Geometry: see drawing. Coordinates: mm, zero at the bounding-box minimum. Give positions to 0.01 mm unless a question says otherwise; leave off trailing zeros. Order: outer loops, then holes, each group sorted by start corner. A loop starts at its lowest first (then second) coordinate and runs counter-clockwise, first axis right, second up. Notation, with made-up numbers: (37, 36.5) - (64, 36.5) arc R15 ccw to (64, 50.5) - close; hole circle Ø9 at (79, 18.5). An arc over 180 degrees is marked (long way). Write each question's results on one line, items separated by ' | '. Start each with the question number.
Item 1: Section A-A on y = 33. Output: boundary loops of the cut face in (x, z).
Item 2: Section B-B on x = 77.5. Output: boundary loops of the cut face in (y, z), and give its area (3 significant figures).
Item 3: Section D-D on y = 15.5. Output: boundary loops of the cut face in (x, z), and give its area (3 significant figures).
Item 4: Contact query for flat-ended pins moving along their axis: pin 1 Ø1.5 at (x, z) = (61, 2.5) entering from +Y; pin 2 Ø1.7 at (x, z) = (99.5, 2) entering from +Y (1 decimal); pin 3 Ø1.7 at (x, z) = (2.5, 2.5) entering from +Y. Output: stop coordinate, or through.
Item 5: Line query: line 1 along X through (y, z) = (41, 1); line 2 along X through (y, z) = (63.5, 0.3); line 3 along Y through (x, z) = (50, 2.1) (1 decimal). Output: solid intervals per line, ascending.
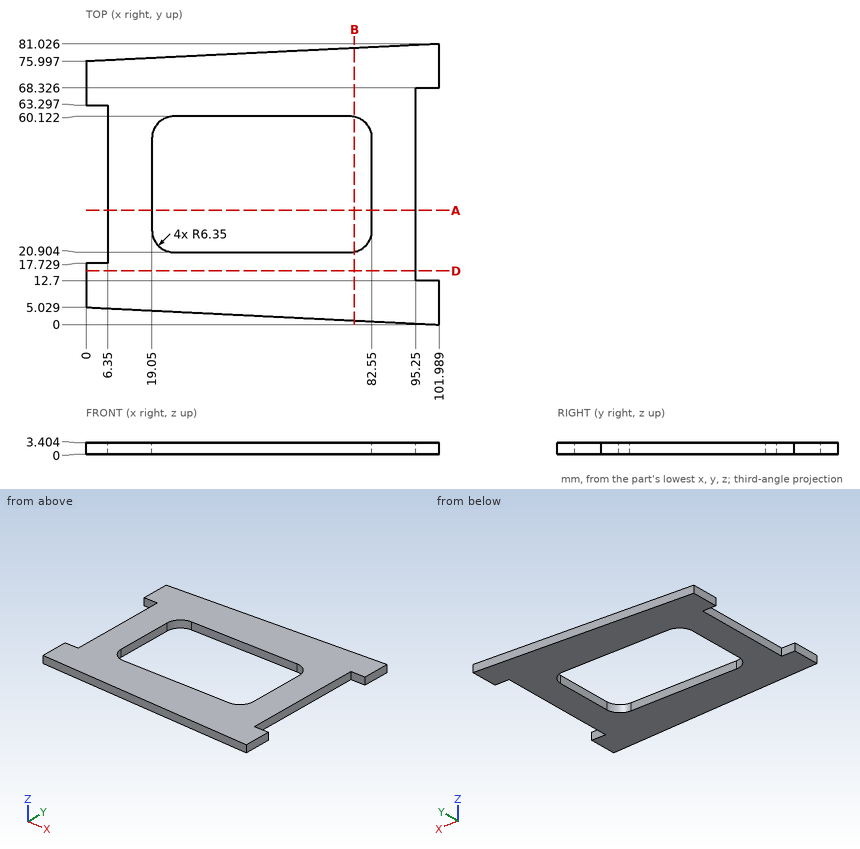
Evaluation:
1) outline: (6.35, 0) - (19.05, 0) - (19.05, 3.4) - (6.35, 3.4) - close; (82.55, 0) - (95.25, 0) - (95.25, 3.4) - (82.55, 3.4) - close
2) outline: (1.21, 0) - (21.04, 0) - (21.04, 3.4) - (1.21, 3.4) - close; (59.99, 0) - (79.82, 0) - (79.82, 3.4) - (59.99, 3.4) - close | area: 135 mm^2
3) outline: (0, 0) - (95.25, 0) - (95.25, 3.4) - (0, 3.4) - close | area: 324 mm^2
4) pin 1: stops at y = 79.04 | pin 2: stops at y = 80.9 | pin 3: stops at y = 76.16
5) line 1: x = 6.35 to 19.05, 82.55 to 95.25 | line 2: x = 0 to 95.25 | line 3: y = 2.6 to 20.9, 60.1 to 78.5
